Print and shaded views of the part. All mm, measured from the part's lowest x, y and z. A direction names the side the tool comes from. Coordinates: 2 decimals unless noted, no trailing zeros. Loops run counter-clockwise (first coordinate to the right, second up) from the corner with the lowest first, then second, coordinate; pieces in that order, holes last. Notation, with made-up numbers: M -9,84.25 L 30,84.25 A33 ccw 30,114.25 Z; hole C -18,-26.5 d6. An arc over 180 degrees is marked long. Answer as a JSON object with one key per item and string values. Group by question number.
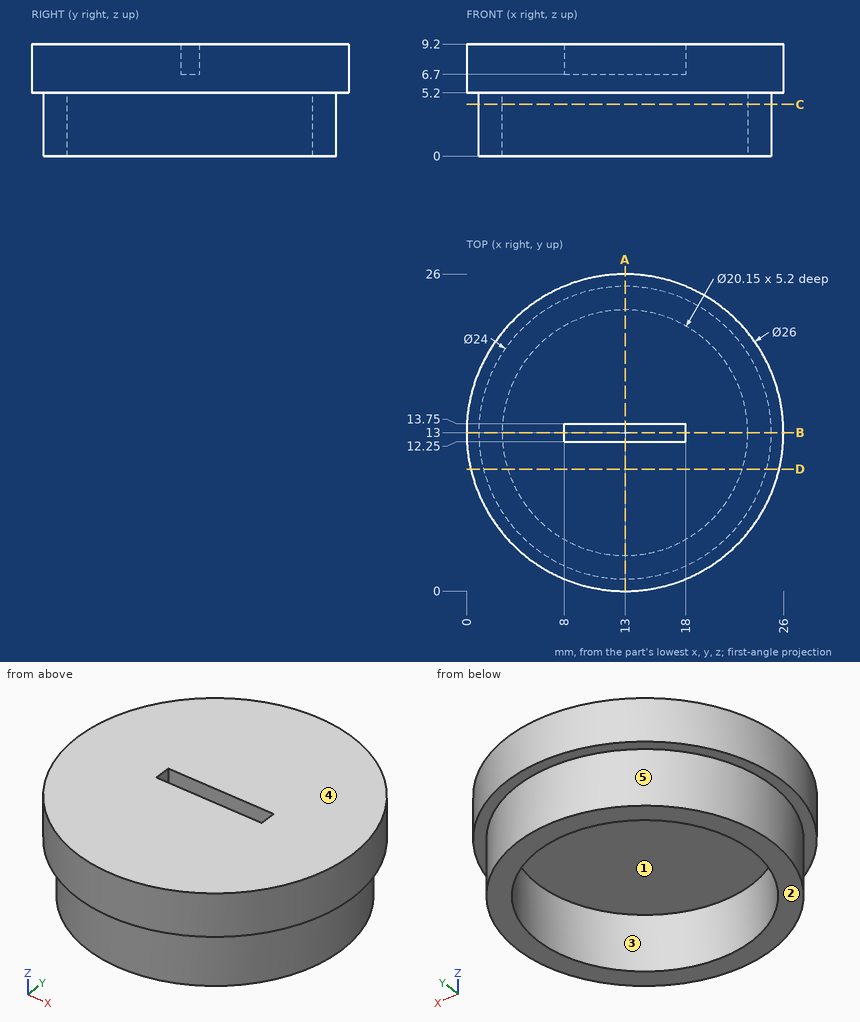
Item 1: Slice it at C-C, the plane z = 4.25. Write the cut outline in (x, y) (3 decimals).
Item 2: Slice it at B-B, the plane y = 13. Write the cut outline in (x, z) (3 decimals).
Item 3: Drill centre lines: L1, parallel to Y at x = 13, z = 1.4 (3 decimals); L2, parallel to X at y = 25, z = 5.5; L3, parallel to Z at x = 10.75, y = 16.5. Where is each one in solid material? Low to high. Write a range as from..to.
Item 4: Pin check, flat tips, straight feed: pin 1 (1 mm diameter, centred on y = 13, z = 1.5, fed in from -X); pin 2 (0.8 mm diameter, centred on x = 11.5, z = 8, fed in from -Y); pin 3 (3 mm diameter, centred on y = 9.5, z = 7, fed in from +X). Stop position of each tip, or through.
Item 5: Tool access for the marked faces 1 and 2: list every direction of +Z, -Z, +X, -X, +Y, -Y with a clear straight run to the whole face (end or side of a thin tool).
Item 6: Slice it at D-D, the plane y = 10. Write the cut outline in (x, z).
Item 7: Slice it at A-A, the plane x = 13. Write the cut outline in (y, z) (3 decimals), then the cut area to 3 significant figures.
Item 8: Pull direction Y, two halves, no side cores. Call the marked faces 3, 4 and 5: released by +Y, released by -Y, zero draft, split by the parting line, or undercut.
Computed:
{
 "1": {"outline": "C 13,13 d24; hole C 13,13 d20.15"},
 "2": {"outline": "M 0,5.2 L 1,5.2 L 1,0 L 2.925,0 L 2.925,5.2 L 23.075,5.2 L 23.075,0 L 25,0 L 25,5.2 L 26,5.2 L 26,9.2 L 18,9.2 L 18,6.7 L 8,6.7 L 8,9.2 L 0,9.2 Z"},
 "3": {"L1": "1..2.925, 23.075..25", "L2": "8..18", "L3": "5.2..9.2"},
 "4": {"pin 1": "x = 1", "pin 2": "y = 0.05", "pin 3": "x = 25.85"},
 "5": {"face 1": "-Z", "face 2": "-Z, +X, -X, +Y, -Y"},
 "6": {"outline": "M 0.35,5.2 L 1.38,5.2 L 1.38,0 L 3.38,0 L 3.38,5.2 L 22.62,5.2 L 22.62,0 L 24.62,0 L 24.62,5.2 L 25.65,5.2 L 25.65,9.2 L 0.35,9.2 Z"},
 "7": {"outline": "M 0,5.2 L 1,5.2 L 1,0 L 2.925,0 L 2.925,5.2 L 23.075,5.2 L 23.075,0 L 25,0 L 25,5.2 L 26,5.2 L 26,9.2 L 13.75,9.2 L 13.75,6.7 L 12.25,6.7 L 12.25,9.2 L 0,9.2 Z", "area": "120 mm2"},
 "8": {"face 3": "undercut", "face 4": "zero draft", "face 5": "split by the parting line"}
}
